Design review of the part built by this model. Coordinates are the model's own, in mm. Coordinates: 2 decimals unless noted, no trailing zeros. Write each loop counter-clockwise with the first axis right and the second up, starting at its lowest first coordinate (ties: lowest second). Pieces come first, ordered by that corner, then holes. Notation, with made-up numbers: (84, 63.5) - (100, 63.5) arc R36 cw to (100, 101.5) - close; hole circle Ø3 at (-6.5, 24.5). An arc over 180 degrees is marked (long way). One line per item, written item: value.
from build123d import *

# Parameters (mm, degrees)
F0_R     = 35.1091
F0_R_2   = 11.393161
F1_DEPTH = 25.4


with BuildPart() as f1:
    # F0 (on Top) → F1 (new body)
    with BuildSketch(Plane.XY):
        with Locations((37.455708, 38.188457)):
            Circle(F0_R)
        with BuildLine():
            ThreePointArc((67.146141, 46.00208), (37.534716, 7.487183), (7.725452, 45.849163))
            Line((7.725452, 45.849163), (11.313939, 43.919829))
            ThreePointArc((11.313939, 43.919829), (14.374897, 24.641617), (29.714165, 12.569925))
            Line((29.714165, 12.569925), (34.466456, 23.405907))
            ThreePointArc((34.466456, 23.405907), (37.000848, 23.113561), (39.548255, 23.252572))
            Line((39.548255, 23.252572), (44.618947, 12.402246))
            ThreePointArc((44.618947, 12.402246), (60.539008, 24.645859), (63.459597, 44.516053))
            Line((63.459597, 44.516053), (67.146141, 46.00208))
        make_face(mode=Mode.SUBTRACT)
        with BuildLine():
            Line((46.820656, 17.996635), (43.649702, 24.437317))
            ThreePointArc((43.649702, 24.437317), (52.493895, 37.042883), (45.661202, 50.842677))
            Line((45.661202, 50.842677), (49.541016, 56.87956))
            ThreePointArc((49.541016, 56.87956), (52.018121, 55.021404), (54.213368, 52.837444))
            Line((54.213368, 52.837444), (57.641099, 55.760898))
            ThreePointArc((57.641099, 55.760898), (36.95968, 64.946534), (16.63291, 55.000709))
            Line((16.63291, 55.000709), (19.981425, 51.974734))
            ThreePointArc((19.981425, 51.974734), (22.082703, 54.284503), (24.486543, 56.27748))
            Line((24.486543, 56.27748), (28.400993, 50.249617))
            ThreePointArc((28.400993, 50.249617), (22.415419, 37.070808), (30.283139, 24.921443))
            Line((30.283139, 24.921443), (27.216956, 18.425362))
            ThreePointArc((27.216956, 18.425362), (16.591173, 30.437125), (16.797069, 46.472938))
            Line((16.797069, 46.472938), (9.129374, 50.028783))
            ThreePointArc((9.129374, 50.028783), (37.314565, 68.889509), (65.671979, 50.288727))
            Line((65.671979, 50.288727), (58.045574, 46.642415))
            ThreePointArc((58.045574, 46.642415), (58.179315, 30.067862), (46.820656, 17.996635))
        make_face(mode=Mode.SUBTRACT)
        with BuildLine():
            ThreePointArc((41.770592, 52.639796), (37.016011, 53.263804), (32.305881, 52.363742))
            Line((32.305881, 52.363742), (28.448893, 58.542554))
            ThreePointArc((28.448893, 58.542554), (36.911639, 60.439659), (45.456988, 58.958423))
            Line((45.456988, 58.958423), (41.770592, 52.639796))
        make_face(mode=Mode.SUBTRACT)
        with Locations((37.455708, 38.188457)):
            Circle(F0_R_2, mode=Mode.SUBTRACT)
    extrude(amount=F1_DEPTH)


solid = f1.part
1. Wall thickness on line 1 along X through (y, z) = (37.5, 2.5); line 2 along Y through (x, z) = (20.5, 8.5); line 3 along Y through (x, z) = (14, 15.75): over which ranges is each line inside the solid? List them lowest first.
Answer block:
line 1: x = 2.35 to 6.76, 10.7 to 15.21, 22.39 to 26.08, 48.83 to 52.52, 59.7 to 64.21, 68.15 to 72.56
line 2: y = 7.45 to 12.59, 17.48 to 23.77, 52.61 to 58.89, 63.78 to 68.93
line 3: y = 12.06 to 18.38, 25.3 to 47.77, 58 to 64.31
2. Mouldability with a two-part tool opening along Y and no side actions: class faces 1 (the face through (22.1, 54.3, 12.5)), 2 (the face through (29.2, 46.5, 25.4)) as released by +Y, released by -Y, zero draft, split by the parting line, or undercut.
Answer block:
face 1: undercut
face 2: zero draft
3. Consider section D-D, the plane y = 66. Write out the cut boundary in (x, z), then the cut area to 3 significant figures.
Answer block:
outline: (16.03, 0) - (24.45, 0) - (24.45, 25.4) - (16.03, 25.4) - close; (50.46, 0) - (58.88, 0) - (58.88, 25.4) - (50.46, 25.4) - close
area: 428 mm^2
4. Consider section A-A, the plane x = 36.5. Write out the cut boundary in (y, z), then the cut area to 3 significant figures.
Answer block:
outline: (3.09, 0) - (7.5, 0) - (7.5, 25.4) - (3.09, 25.4) - close; (23.14, 0) - (26.84, 0) - (26.84, 25.4) - (23.14, 25.4) - close; (49.54, 0) - (53.24, 0) - (53.24, 25.4) - (49.54, 25.4) - close; (60.43, 0) - (64.93, 0) - (64.93, 25.4) - (60.43, 25.4) - close; (68.87, 0) - (73.28, 0) - (73.28, 25.4) - (68.87, 25.4) - close
area: 526 mm^2
5. Consider section C-C, the plane z = 10.5. Give the number of separate pieces and of enclosed holes in the cut face, then the cut area to 3 significant figures.
Answer block:
separate pieces: 1
enclosed holes: 4
area: 1,950 mm^2
6. Insertion check: pin 1 Ø8 at (x, z) = (29.5, 15) entering from +Y; pin 2 Ø1.5 at (x, z) = (47.5, 3) entering from -Y; pin 3 Ø1.5 at (y, z) = (44, 21.5) entering from +X; pin 4 Ø13.5 at (x, y) = (37.46, 38.19) entering from +Z. Each pin has a flat end and moves straight along its axis. Give the tip position at first contact, or say it passes through.
Answer block:
pin 1: stops at y = 73.07
pin 2: stops at y = 4.33
pin 3: stops at x = 72.2
pin 4: passes through
7. Consider section B-B, the plane y = 9.5. Write out the cut boundary in (x, z).
Answer block:
outline: (17.22, 0) - (26.52, 0) - (26.52, 25.4) - (17.22, 25.4) - close; (48.39, 0) - (57.69, 0) - (57.69, 25.4) - (48.39, 25.4) - close
